```python
from build123d import *

# Parameters (mm, degrees)
SKETCH_1_W          = 800
SKETCH_1_H          = 800
SKETCH_1_W_2        = 385
SKETCH_1_H_2        = 780
EXTRUDE_1_DEPTH     = 200
SKETCH_2_W          = 800
SKETCH_2_H          = 800
EXTRUDE_2_DEPTH     = 10
EXTRUDE_3_DEPTH     = 10
EXTRUDE_3_2_DEPTH   = 10
SKETCH_4_R          = 4
CUT_EXTRUDE_1_DEPTH = 10
SKETCH_5_R          = 4
CUT_EXTRUDE_2_DEPTH = 10
EXTRUDE_4_DEPTH     = 10
CUT_EXTRUDE_3_REACH = 1087.28
SKETCH_7_R          = 4
CUT_EXTRUDE_4_REACH = 1156.96
SKETCH_8_R          = 4
SKETCH_9_W          = 2800
SKETCH_9_H          = 2800
SKETCH_9_W_2        = 800
SKETCH_9_H_2        = 800
CUT_EXTRUDE_5_DEPTH = 1157.647305275


with BuildPart() as part:
    # Sketch 1 → Extrude 1 (new body)
    with BuildSketch(Plane(origin=(0, 0, 0), x_dir=(1, 0, 0), z_dir=(0, 1, 0))):
        Rectangle(SKETCH_1_W, SKETCH_1_H)
        with Locations((-197.5, 0)):
            Rectangle(SKETCH_1_W_2, SKETCH_1_H_2, mode=Mode.SUBTRACT)
        with Locations((197.5, 0)):
            Rectangle(SKETCH_1_W_2, SKETCH_1_H_2, mode=Mode.SUBTRACT)
    extrude(amount=EXTRUDE_1_DEPTH)

    # Sketch 2 → Extrude 2 (add)
    with BuildSketch(Plane.XZ):
        Rectangle(SKETCH_2_W, SKETCH_2_H)
    extrude(amount=-EXTRUDE_2_DEPTH)

    # Sketch 4 → Cut-Extrude 1 (cut)
    with BuildSketch(Plane.ZY.offset(400)):
        with Locations((180, 160)):
            Circle(SKETCH_4_R)
        with Locations((200, 160)):
            Circle(SKETCH_4_R)
        with Locations((-20, 160)):
            Circle(SKETCH_4_R)
        with Locations((0, 160)):
            Circle(SKETCH_4_R)
    cut_extrude_1 = extrude(amount=-CUT_EXTRUDE_1_DEPTH, mode=Mode.SUBTRACT)


with BuildPart() as body_2:
    # Sketch 3 → Extrude 3 (new body)
    with BuildSketch(Plane(origin=(0, 200, 0), x_dir=(1, 0, 0), z_dir=(0, 1, 0))):
        with BuildLine():
            Line((-400, 400), (-400, -400))
            Line((-400, -400), (-552.7864045, -400))
            ThreePointArc((-552.7864045, -400), (-682.754282993, -327.538161854), (-689.4427191, -178.8854382))
            Line((-689.4427191, -178.8854382), (-400, 400))
        make_face()
    extrude(amount=-EXTRUDE_3_DEPTH)

    # Sketch 5 → Cut-Extrude 2 (cut)
    with BuildSketch(Plane(origin=(0, 200, 0), x_dir=(1, 0, 0), z_dir=(0, 1, 0))):
        with Locations(Location((-430, -180, 0), (0, 0, 270))):
            Circle(SKETCH_5_R)
        with Locations(Location((-430, -200, 0), (0, 0, 270))):
            Circle(SKETCH_5_R)
        with Locations(Location((-430, 20, 0), (0, 0, 270))):
            Circle(SKETCH_5_R)
        with Locations(Location((-430, 0, 0), (0, 0, 270))):
            Circle(SKETCH_5_R)
    cut_extrude_2 = extrude(amount=-CUT_EXTRUDE_2_DEPTH, mode=Mode.SUBTRACT)


with BuildPart() as body_3:
    # Sketch 3 → Extrude 3 2 (new body)
    with BuildSketch(Plane(origin=(0, 200, 0), x_dir=(1, 0, 0), z_dir=(0, 1, 0))):
        with BuildLine():
            Line((689.4427191, -178.8854382), (400, 400))
            Line((400, 400), (400, -400))
            Line((400, -400), (552.7864045, -400))
            ThreePointArc((552.7864045, -400), (682.754282993, -327.538161854), (689.4427191, -178.8854382))
        make_face()
    extrude(amount=-EXTRUDE_3_2_DEPTH)


with BuildPart() as mirror_1_tool:
    # Mirror 1: Cut-Extrude 1, Cut-Extrude 2 across plane
    add(cut_extrude_1.mirror(Plane(origin=(0, 0, 0), x_dir=(0, 0, 1), z_dir=(1, 0, 0))))
    add(cut_extrude_2.mirror(Plane(origin=(0, 0, 0), x_dir=(0, 0, 1), z_dir=(1, 0, 0))))


with BuildPart() as part_1:
    add(part.part)

    # Mirror 1: cut by mirror_1_tool
    add(mirror_1_tool.part, mode=Mode.SUBTRACT)


    add(body_2.part)  # Extrude 4 merges body 2


with BuildPart() as body_3_1:
    add(body_3.part)

    # Mirror 1: cut by mirror_1_tool
    add(mirror_1_tool.part, mode=Mode.SUBTRACT)


with BuildPart() as part_2:
    add(part_1.part)

    add(body_3_1.part)  # Extrude 4 merges body 3
    # Sketch 6 → Extrude 4 (add)
    with BuildSketch(Plane(origin=(0, 200, 0), x_dir=(1, 0, 0), z_dir=(0, 1, 0))):
        with BuildLine():
            Line((-400, 400), (-221.1145618, 757.7708764))
            ThreePointArc((-221.1145618, 757.7708764), (0, 894.427191), (221.1145618, 757.7708764))
            Line((221.1145618, 757.7708764), (400, 400))
            Line((400, 400), (-400, 400))
        make_face()
    extrude(amount=-EXTRUDE_4_DEPTH)

    # Sketch 7 → Cut-Extrude 3 (cut, up to next)
    with BuildSketch(Plane(origin=(0, 0, -400), x_dir=(-1, 0, 0), z_dir=(0, 0, -1)), mode=Mode.PRIVATE) as cut_extrude_3_sk1:
        with Locations((-200, 160)):
            Circle(SKETCH_7_R)
    cut_extrude_3_tool1 = extrude(cut_extrude_3_sk1.sketch, amount=-CUT_EXTRUDE_3_REACH, mode=Mode.PRIVATE) & part_2.part
    # Sketch 7 → Cut-Extrude 3 (cut, up to next)
    with BuildSketch(Plane(origin=(0, 0, -400), x_dir=(-1, 0, 0), z_dir=(0, 0, -1)), mode=Mode.PRIVATE) as cut_extrude_3_sk2:
        with Locations((-180, 160)):
            Circle(SKETCH_7_R)
    cut_extrude_3_tool2 = extrude(cut_extrude_3_sk2.sketch, amount=-CUT_EXTRUDE_3_REACH, mode=Mode.PRIVATE) & part_2.part
    cut_extrude_3_1 = cut_extrude_3_tool1.solids().sort_by_distance((200, 160, -400))[0]
    add(cut_extrude_3_1, mode=Mode.SUBTRACT)
    cut_extrude_3_2 = cut_extrude_3_tool2.solids().sort_by_distance((180, 160, -400))[0]
    add(cut_extrude_3_2, mode=Mode.SUBTRACT)
    cut_extrude_3 = cut_extrude_3_1 + cut_extrude_3_2  # Cut-Extrude 3 as one shape, for the pattern or mirror that repeats it

    # Sketch 8 → Cut-Extrude 4 (cut, up to next)
    with BuildSketch(Plane.XZ.offset(-190), mode=Mode.PRIVATE) as cut_extrude_4_sk1:
        with Locations(Location((180, -430, 0), (0, 0, 270))):
            Circle(SKETCH_8_R)
    cut_extrude_4_tool1 = extrude(cut_extrude_4_sk1.sketch, amount=-CUT_EXTRUDE_4_REACH, mode=Mode.PRIVATE) & part_2.part
    # Sketch 8 → Cut-Extrude 4 (cut, up to next)
    with BuildSketch(Plane.XZ.offset(-190), mode=Mode.PRIVATE) as cut_extrude_4_sk2:
        with Locations(Location((200, -430, 0), (0, 0, 270))):
            Circle(SKETCH_8_R)
    cut_extrude_4_tool2 = extrude(cut_extrude_4_sk2.sketch, amount=-CUT_EXTRUDE_4_REACH, mode=Mode.PRIVATE) & part_2.part
    cut_extrude_4_1 = cut_extrude_4_tool1.solids().sort_by_distance((180, 190, -430))[0]
    add(cut_extrude_4_1, mode=Mode.SUBTRACT)
    cut_extrude_4_2 = cut_extrude_4_tool2.solids().sort_by_distance((200, 190, -430))[0]
    add(cut_extrude_4_2, mode=Mode.SUBTRACT)
    cut_extrude_4 = cut_extrude_4_1 + cut_extrude_4_2  # Cut-Extrude 4 as one shape, for the pattern or mirror that repeats it

    # Mirror 2: Cut-Extrude 3, Cut-Extrude 4 across plane
    add(cut_extrude_3.mirror(Plane(origin=(0, 0, 0), x_dir=(0, 0, 1), z_dir=(1, 0, 0))), mode=Mode.SUBTRACT)
    add(cut_extrude_4.mirror(Plane(origin=(0, 0, 0), x_dir=(0, 0, 1), z_dir=(1, 0, 0))), mode=Mode.SUBTRACT)

    # Sketch 9 → Cut-Extrude 5 (cut, through all)
    with BuildSketch(Plane.XZ):
        Rectangle(SKETCH_9_W, SKETCH_9_H)
        Rectangle(SKETCH_9_W_2, SKETCH_9_H_2, mode=Mode.SUBTRACT)
    extrude(amount=-CUT_EXTRUDE_5_DEPTH, mode=Mode.SUBTRACT)


solid = part_2.part
```
Geometry check sheet. Reference: the model listing, model coordinates, mm. A direction names the side the tool comes from. Round coordinates to 2 decimals unless told otherwise and drop trailing zeros. Write each loop counter-clockwise with the first axis right and the second up, starting at its lowest first coordinate (ties: lowest second). Pieces come first, ordered by that corner, then holes. Notation, with made-up numbers: (-30.5, 83.25) -> (22.5, 83.25) arc R35 ccw to (22.5, 115.25) -> close; hole circle Ø3 at (63.25, 20). An arc over 180 degrees is marked (long way). Put each result on its own line as item: value.
1) Depth check by flat-ended pin: P1, Ø6.5, axis at y = 160, z = 200, coming from the -X side; P2, Ø5, axis at x = -200, y = 160, coming from the -Z side; P3, Ø6.5, axis at y = 160, z = 0, coming from the +X side. Enter the tip coordinate at first touch or a pass-through.
Recorded:
P1: stops at x = -5
P2: stops at z = 390
P3: stops at x = 5
2) Release check for a two-part mould opening along X. For faces 1 (the face through (-6, 99, -400)), 2 (the face through (-5, 104, 5)), 3 (the face through (-400, 99, -6)) record: pulls with the +X half, pulls with the -X half, needs draft (parallel to the pull), parting line crosses it, or undercut.
Recorded:
face 1: needs draft
face 2: undercut
face 3: pulls with the -X half
3) Thickness scan on probe 1 along X at (y, z) = (134, -89.5); probe 2 along Y at (x, z) = (180, -395.75); probe 3 along Z at (x, y) = (359, 156). Record the ranges inside material, lowest first. Write a range as from..to.
Recorded:
probe 1: x = -400..-390, -5..5, 390..400
probe 2: y = 0..156, 164..200
probe 3: z = -400..-390, 390..400
4) Cross-section at B-B, the plane y = 48.5. Enter the section's corners in (x, z).
Recorded:
outline: (-400, -400) -> (400, -400) -> (400, 400) -> (-400, 400) -> close; hole (-390, -390) -> (-5, -390) -> (-5, 390) -> (-390, 390) -> close; hole (5, -390) -> (390, -390) -> (390, 390) -> (5, 390) -> close
5) Cross-section at A-A, the plane z = 166. Enter the section's corners in (x, y), plus the area to 3 significant figures.
Recorded:
outline: (-400, 0) -> (400, 0) -> (400, 200) -> (390, 200) -> (390, 10) -> (5, 10) -> (5, 200) -> (-5, 200) -> (-5, 10) -> (-390, 10) -> (-390, 200) -> (-400, 200) -> close
area: 13,700 mm2
6) Cross-section at C-C, the plane x = -307. Enter the section's corners in (y, z).
Recorded:
outline: (0, -400) -> (200, -400) -> (200, -390) -> (10, -390) -> (10, 390) -> (200, 390) -> (200, 400) -> (0, 400) -> close
7) Access from +Z, -Z, +X, -X, +Y, -Y to the whole of each face (thin tool, end or side, straight path). Record for faces 4 (the face through (-6, 101, 400)), 5 (the face through (195, 104, -390)).
Recorded:
face 4: +Z, +X, -X, +Y, -Y
face 5: +Y
